The listing builds one solid part. Answer for the finished solid, in the listing's coordinates (mm). A direction names the side the tool comes from. Coordinates: 2 decimals unless noted, no trailing zeros. Loops run counter-clockwise (first coordinate to the right, second up) from the corner with the lowest first, then second, coordinate; pieces in that order, holes last. Notation, with made-up numbers: M 14.25,-1.75 L 37.25,-1.75 A9 cw 37.25,2.25 Z; hole C 58,77 d8. An arc over 180 degrees is marked long. Return JSON: item names as keys, results as strings. Group by question number.
1. Section B-B (x = 6.74) is taken. Write down the section's boundary in (y, z).
2. Section D-D (x = 14.25) is taken. Write down the section's boundary in (y, z), then the cut area to 3 significant figures.
3. Given P1, Ø4, axis at x = 9.5, y = 4.5, coming from the -Z side; P2, Ø1.5, axis at x = 7.5, y = 3, coming from the +Z side; P3, Ø1.7, axis at y = 3.5, z = 3.5, coming from the -X side, each flat-ended and moving along its own axis, determine where each tip first touches the part or whether it passes through.
4. Straight lines are drawn through the part: L1, parallel to Y at x = 24.5, z = 3.4; L2, parallel to Y at x = 6.74, z = -2.7; L3, parallel to X at y = 3.75, z = -10. For each, find the intervals that lie inside material, in ascending order. Write a range as from..to.
5. Which of the six approach directions +Z, -Z, +X, -X, +Y, -Y give full straight-line access (tool end or side, diameter ignored) to faces 1 (the face through (3.64, 6, -8)), 2 (the face through (5.08, 7.52, -0.75)), 3 (the face through (11, 6, 0))?
6. The mould has two halves that part along Z. Classify faces 4 (the face through (23.99, 7, 4)), 5 (the face through (13, 11.5, -2)), 6 (the face through (2, 6, -12.8)): pulls with the +Z half, pulls with the -Z half, needs draft (parallel to the pull), parting line crosses it, or undercut.
7. Section A-A (z = 3.4) is taken. Write down the section's boundary in (x, y), then the cut area to 3 significant figures.
8. Section C-C (z = -2) is taken. Write down the section's boundary in (x, y).
```python
from build123d import *

# Parameters (mm, degrees)
BOSS_EXTRUDE1_DEPTH = 11.5
SKETCH4_R           = 1.5
CUT_EXTRUDE1_DEPTH  = 4.5
SKETCH5_R           = 2.25
CUT_EXTRUDE2_DEPTH  = 1.5
SKETCH6_R           = 2.15
CUT_EXTRUDE3_DEPTH  = 1.75
SKETCH7_R           = 1.15
CUT_EXTRUDE4_DEPTH  = 2.5
FILLET4_R           = 0.5
FILLET5_R           = 0.5
FILLET6_R           = 0.5


with BuildPart() as part:
    # Sketch1 → Boss-Extrude1 (new body)
    with BuildSketch(Plane(origin=(0, 0, 0), x_dir=(1, 0, 0), z_dir=(0, 1, 0))):
        Polygon((0, 0), (0, 12.8), (3.64, 12.8), (3.64, 4), (26.24, 4), (26.24, -6.8), (22.24, -6.8), (22.24, 0), align=None)
    extrude(amount=BOSS_EXTRUDE1_DEPTH)

    # Sketch4 → Cut-Extrude1 (cut)
    with BuildSketch(Plane.XY):
        with Locations((6.74, 6)):
            Circle(SKETCH4_R)
    extrude(amount=-CUT_EXTRUDE1_DEPTH, mode=Mode.SUBTRACT)

    # Sketch5 → Cut-Extrude2 (cut)
    with BuildSketch(Plane.XY):
        with Locations((6.74, 6)):
            Circle(SKETCH5_R)
    extrude(amount=-CUT_EXTRUDE2_DEPTH, mode=Mode.SUBTRACT)

    # Sketch6 → Cut-Extrude3 (cut)
    with BuildSketch(Plane.ZY.offset(-22.24)):
        with Locations((3.4, 5.75)):
            Circle(SKETCH6_R)
    extrude(amount=-CUT_EXTRUDE3_DEPTH, mode=Mode.SUBTRACT)

    # Sketch7 → Cut-Extrude4 (cut)
    with BuildSketch(Plane.ZY.offset(-23.99)):
        with Locations((3.4, 5.75)):
            Circle(SKETCH7_R)
    extrude(amount=-CUT_EXTRUDE4_DEPTH, mode=Mode.SUBTRACT)

    # Fillet4
    fillet4_edges = [part.edges().sort_by_distance(p)[0] for p in [
        (4.49, 6, 0),
        (4.49, 6, -1.5),
    ]]
    fillet(fillet4_edges, radius=FILLET4_R)

    # Fillet5
    fillet5_edges = [part.edges().sort_by_distance(p)[0] for p in [
        (23.99, 5.75, 1.25),
        (22.24, 5.75, 1.25),
    ]]
    fillet(fillet5_edges, radius=FILLET5_R)

    # Fillet6
    fillet6_edges = [part.edges().sort_by_distance(p)[0] for p in [
        (24.24, 11.5, 6.8),
        (22.24, 0, 3.4),
        (11.12, 0, 0),
        (0, 5.75, 0),
        (22.24, 5.75, 6.8),
        (22.24, 5.75, 0),
        (0, 11.5, -6.4),
        (11.12, 11.5, 0),
        (22.24, 11.5, 3.4),
        (0, 0, -6.4),
        (24.24, 0, 6.8),
    ]]
    fillet(fillet6_edges, radius=FILLET6_R)


solid = part.part
```
Worked out:
{
 "1": {"outline": "M 0,-4 L 4.5,-4 L 4.5,-1.5 L 4.25,-1.5 A0.5 cw 3.75,-1 L 3.75,-0.5 A0.5 ccw 3.25,0 L 0.5,0 A0.5 ccw 0,-0.5 Z; M 7.5,-4 L 11.5,-4 L 11.5,-0.5 A0.5 ccw 11,0 L 8.75,0 A0.5 ccw 8.25,-0.5 L 8.25,-1 A0.5 cw 7.75,-1.5 L 7.5,-1.5 Z"},
 "2": {"outline": "M 0,-4 L 11.5,-4 L 11.5,-0.5 A0.5 ccw 11,0 L 0.5,0 A0.5 ccw 0,-0.5 Z", "area": "45.9 mm^2"},
 "3": {"P1": "z = -4", "P2": "z = 0", "P3": "x = 22.24"},
 "4": {"L1": "0..4.6, 6.9..11.5", "L2": "0..4.5, 7.5..11.5", "L3": "0..3.64"},
 "5": {"face 1": "-Z, +X, +Y, -Y", "face 2": "+Z", "face 3": "+Z, -X, +Y, -Y"},
 "6": {"face 4": "undercut", "face 5": "needs draft", "face 6": "pulls with the -Z half"},
 "7": {"outline": "M 22.24,0.5 A0.5 ccw 22.74,0 L 26.24,0 L 26.24,4.6 L 23.99,4.6 L 23.99,4.1 A0.5 cw 23.49,3.6 L 22.74,3.6 A0.5 ccw 22.24,3.1 Z; M 22.24,8.4 A0.5 ccw 22.74,7.9 L 23.49,7.9 A0.5 cw 23.99,7.4 L 23.99,6.9 L 26.24,6.9 L 26.24,11.5 L 22.74,11.5 A0.5 ccw 22.24,11 Z", "area": "33.2 mm^2"},
 "8": {"outline": "M 0,0.5 A0.5 ccw 0.5,0 L 26.24,0 L 26.24,11.5 L 0.5,11.5 A0.5 ccw 0,11 Z; hole C 6.74,6 d3"}
}
